```python
from build123d import *

# Parameters (mm, degrees)
SKETCH_1_W                  = 10
SKETCH_1_H                  = 10
EXTRUDE_1_DEPTH             = 17
CUT_EXTRUDE_1_DEPTH         = 13
HOLE_WIZARD_M32_D           = 2.5
HOLE_WIZARD_M32_DEPTH       = 10.5
HOLE_WIZARD_M32_CSINK_D     = 3.3
HOLE_WIZARD_M32_CSINK_ANGLE = 90
HOLE_WIZARD_M32_TIP         = 0.751075774
CHAMFER_1_SIZE              = 1


with BuildPart() as part:
    # Эскиз1 → Бобышка-Вытянуть1 (new body)
    with BuildSketch(Plane.XY):
        with Locations((5, 5)):
            Rectangle(SKETCH_1_W, SKETCH_1_H)
    extrude(amount=EXTRUDE_1_DEPTH)

    # Эскиз7 → Вырез-Вытянуть1 (cut)
    with BuildSketch(Plane.XY.offset(17)):
        Polygon((0.5, 4), (0.5, 10), (0, 10), (0, 0), (10, 0), (10, 4), align=None)
    extrude(amount=-CUT_EXTRUDE_1_DEPTH, mode=Mode.SUBTRACT)

    # Эскиз3 → Отверстие обработанное метчиком M31 (revolve, cut)
    with BuildSketch(Plane(origin=(10, 7, 10.5), x_dir=(0, 0, -1), z_dir=(0, 1, 0))):
        Polygon((0, 0), (0, 9.5), (1.65, 9.5), (1.25, 9.1), (1.25, 0.4), (1.65, 0), align=None)
    revolve(axis=Axis((16.35, 7, 10.5), (-1, 0, 0)), mode=Mode.SUBTRACT)

    # Отверстие обработанное метчиком M32
    with Locations(Plane(origin=(0, 0, 0), x_dir=(-1, 0, 0), z_dir=(0, 0, -1))):
        with Locations((-3, 3), (-7, 7)):
            CounterSinkHole(HOLE_WIZARD_M32_D / 2, HOLE_WIZARD_M32_CSINK_D / 2, depth=HOLE_WIZARD_M32_DEPTH, counter_sink_angle=HOLE_WIZARD_M32_CSINK_ANGLE)
            with Locations((0, 0, -(HOLE_WIZARD_M32_DEPTH + HOLE_WIZARD_M32_TIP / 2))):  # 118° drill point
                Cone(0, HOLE_WIZARD_M32_D / 2, HOLE_WIZARD_M32_TIP, mode=Mode.SUBTRACT)

    # Фаска1
    chamfer_1_edges = [part.edges().sort_by_distance(p)[0] for p in [
        (10, 0, 2),
    ]]
    chamfer(chamfer_1_edges, length=CHAMFER_1_SIZE)


solid = part.part
```
Input: part model. Units: mm. Frame: model coordinates. A direction names the side the tool comes from. Coordinates: 2 decimals unless noted, no trailing zeros. Loops run counter-clockwise (first coordinate to the right, second up) from the corner with the lowest first, then second, coordinate; pieces in that order, holes last. Notation, with made-up numbers: M 21.5,73.5 L 36.5,73.5 A21 ccw 36.5,93.5 Z; hole C 70,-31.75 d5. An arc over 180 degrees is marked long. One line per item, written item: value.
(1) Pull-direction query (Z, two-part tool) for faces 1 (the flat face through (5, 5, 0)), 2 (the flat face through (5, 4, 11)), 3 (the cylindrical face through (5.31, 6.95, 11.75)), 4 (the flat face through (5, 7, 17)); classes: +Z half, -Z half, draft (parallel to the pull), parting line (faces both ways), or undercut.
Filled in:
face 1: -Z half
face 2: draft
face 3: undercut
face 4: +Z half
(2) Section C-C (y = 7). Output: boundary loops of the cut face in (x, z).
Filled in:
outline: M 0,0 L 5.35,0 L 5.75,0.4 L 5.75,9.25 L 0.9,9.25 L 0.5,8.85 L 0.5,4 L 0,4 Z; M 0.5,12.15 L 0.9,11.75 L 9.6,11.75 L 10,12.15 L 10,17 L 0.5,17 Z; M 8.25,0.4 L 8.65,0 L 10,0 L 10,8.85 L 9.6,9.25 L 8.25,9.25 Z
(3) Reachability of faces 5 (the flat face through (0.5, 8, 12)), 6 (the flat face through (9.5, 0.5, 2)), 7 (the cylindrical face through (5.75, 7.05, 5.52)) from +Z, -Z, +X, -X, +Y, -Y: full face, straight path, thin tool, end or side. Return the list, or none.
Filled in:
face 5: +Z, -X, +Y, -Y
face 6: +Z, -Z, +X, -Y
face 7: -Z
(4) Pin query (flat end, axial travel): pin 1 (6 mm diameter, centred on y = 3, z = 8.5, fed in from -X); pin 2 (5 mm diameter, centred on x = 5.5, z = 13, fed in from -Y). Return the tip coordinate at first contact, or that it passes through.
Filled in:
pin 1: x = 0.5
pin 2: y = 4
(5) Line query: line 1 along X through (y, z) = (7, 7); line 2 along Y through (x, z) = (4.5, 10.5); line 3 along X through (y, z) = (2, 3.5). Output: solid intervals per line, ascending. Write a range as from..to.
Filled in:
line 1: 0.5..5.75, 8.25..10
line 2: 4..5.75, 8.25..10
line 3: 0..2.25, 3.75..10
(6) Section A-A (y = 3). Output: boundary loops of the cut face in (x, z), and give its area (3 significant figures).
Filled in:
outline: M 0,0 L 1.35,0 L 1.75,0.4 L 1.75,4 L 0,4 Z; M 4.25,0.4 L 4.65,0 L 10,0 L 10,4 L 4.25,4 Z
area: 29.8 mm^2
(7) Section B-B (x = 3). Output: boundary loops of the cut face in (y, z), and give its area (3 significant figures).
Filled in:
outline: M 0,0 L 1.35,0 L 1.75,0.4 L 1.75,4 L 0,4 Z; M 4,10.65 L 4.25,10.5 L 4.25,0.4 L 4.65,0 L 10,0 L 10,17 L 4,17 Z; hole C 7,10.5 d2.5
area: 101 mm^2
(8) Section D-D (z = 5). Output: boundary loops of the cut face in (x, y).
Filled in:
outline: M 0.5,4 L 2.25,4 A1.25 cw 3.75,4 L 10,4 L 10,10 L 0.5,10 Z; hole C 7,7 d2.5
